CAD build for the part. Positions are in the model's coordinates, mm. Face numbers are marked on the shaded views. A direction names the side the tool comes from. Give positions to 0.01 mm unless a question says otherwise; leave off trailing zeros. Loops run counter-clockwise (first coordinate to the right, second up) from the corner with the lowest first, then second, coordinate; pieces in that order, holes last. Notation, with made-up numbers: (33.5, -8) -> (87.5, -8) arc R17 cw to (87.5, 5) -> close; hole circle Ø1 at (69, 15). An arc over 180 degrees is marked (long way). Use one line per item in the form item = value.
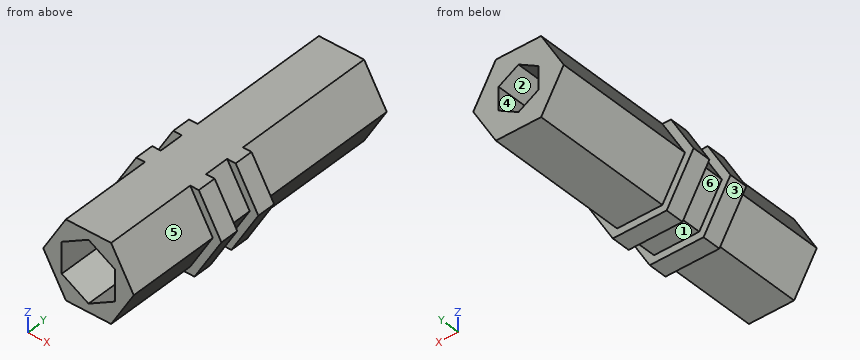
Autodesk Inventor part; units mm, degrees
ref_plane "YZ Plane" through (0, 0, 0) normal (1, 0, 0) x (0, 1, 0)
ref_plane "XZ Plane" through (0, 0, 0) normal (0, 1, 0) x (-1, 0, 0)
ref_plane "XY Plane" through (0, 0, 0) normal (0, 0, 1) x (1, 0, 0)
sketch "Sketch2" plane through (0, 0, 0) normal (0, 1, 0) x (-1, 0, 0)
  line L0 (3.6373, 0) -> (1.8187, -3.15)
  line L1 (1.8187, -3.15) -> (-1.8187, -3.15)
  line L2 (-1.8187, -3.15) -> (-3.6373, 0)
  line L3 (-3.6373, 0) -> (-1.8187, 3.15)
  line L4 (-1.8187, 3.15) -> (1.8187, 3.15)
  line L5 (1.8187, 3.15) -> (3.6373, 0)
  point P0 (0, 0)
  point P1 (0, 0)
  dimension "d0" = 6.3
extrude "Joint End" add sketch "Sketch2" along normal blind 7.5
sketch "Sketch3" plane through (0, 7.5, 0) normal (0, 1, 0) x (1, 0, 0)
  line L0 (4.3301, 0) -> (2.1651, -3.75)
  line L1 (2.1651, -3.75) -> (-2.1651, -3.75)
  line L2 (-2.1651, -3.75) -> (-4.3301, 0)
  line L3 (-4.3301, 0) -> (-2.1651, 3.75)
  line L4 (-2.1651, 3.75) -> (2.1651, 3.75)
  line L5 (2.1651, 3.75) -> (4.3301, 0)
  point P0 (0, 0)
  point P1 (0, 0)
  dimension "d3" = 7.5
extrude "Spring Stop 1" add sketch "Sketch3" along normal blind 1.5
sketch "Sketch4" plane through (0, 9, 0) normal (0, 1, 0) x (1, 0, 0)
  line L0 (3.6373, 0) -> (1.8187, -3.15)
  line L1 (1.8187, -3.15) -> (-1.8187, -3.15)
  line L2 (-1.8187, -3.15) -> (-3.6373, 0)
  line L3 (-3.6373, 0) -> (-1.8187, 3.15)
  line L4 (-1.8187, 3.15) -> (1.8187, 3.15)
  line L5 (1.8187, 3.15) -> (3.6373, 0)
  point P0 (0, 0)
  point P1 (0, 0)
  point P2 (0, 0)
  dimension "d6" = 6.3
extrude "Spring Slot" add sketch "Sketch4" along normal blind 2
sketch "Sketch5" plane through (0, 11, 0) normal (0, 1, 0) x (1, 0, 0)
  line L0 (4.3301, 0) -> (2.1651, -3.75)
  line L1 (2.1651, -3.75) -> (-2.1651, -3.75)
  line L2 (-2.1651, -3.75) -> (-4.3301, 0)
  line L3 (-4.3301, 0) -> (-2.1651, 3.75)
  line L4 (-2.1651, 3.75) -> (2.1651, 3.75)
  line L5 (2.1651, 3.75) -> (4.3301, 0)
  point P0 (0, 0)
  point P1 (0, 0)
  dimension "d9" = 7.5
extrude "Spring Stop 2" add sketch "Sketch5" along normal blind 1.5
sketch "Sketch6" plane through (0, 12.5, 0) normal (0, 1, 0) x (1, 0, 0)
  line L0 (3.6373, 0) -> (1.8187, -3.15)
  line L1 (1.8187, -3.15) -> (-1.8187, -3.15)
  line L2 (-1.8187, -3.15) -> (-3.6373, 0)
  line L3 (-3.6373, 0) -> (-1.8187, 3.15)
  line L4 (-1.8187, 3.15) -> (1.8187, 3.15)
  line L5 (1.8187, 3.15) -> (3.6373, 0)
  point P0 (0, 0)
  point P1 (0, 0)
  dimension "d12" = 6.3
extrude "Carbon End" add sketch "Sketch6" along normal blind 11.5
sketch "Sketch10" plane through (0, 0, 0) normal (0, -1, 0) x (1, 0, 0)
  line L0 (0, -2.4826) -> (-2.15, -1.2413)
  line L1 (-2.15, -1.2413) -> (-2.15, 1.2413)
  line L2 (-2.15, 1.2413) -> (0, 2.4826)
  line L3 (0, 2.4826) -> (2.15, 1.2413)
  line L4 (2.15, 1.2413) -> (2.15, -1.2413)
  line L5 (2.15, -1.2413) -> (0, -2.4826)
  point P0 (0, 0)
  point P1 (0, 0)
  dimension "d27" = 4.3
extrude "Arm Hole" cut sketch "Sketch10" against normal blind 10
sketch "Sketch11" plane through (0, 24, 0) normal (0, 1, 0) x (1, 0, 0)
  line L0 (0, -1.8475) -> (-1.6, -0.9238)
  line L1 (-1.6, -0.9238) -> (-1.6, 0.9238)
  line L2 (-1.6, 0.9238) -> (0, 1.8475)
  line L3 (0, 1.8475) -> (1.6, 0.9238)
  line L4 (1.6, 0.9238) -> (1.6, -0.9238)
  line L5 (1.6, -0.9238) -> (0, -1.8475)
  point P0 (0, 0)
  point P1 (0, 0)
  dimension "d30" = 3.2
  dimension "d31" = 3.695
extrude "Carbon Hole" cut sketch "Sketch11" against normal blind 10
sketch "Sketch12" plane through (0, 12.5, 0) normal (0, 1, 0) x (1, 0, 0)
  line L0 (2.1651, -3.75) -> (4.3301, 0)
  line L1 (-4.3301, 0) -> (-2.1651, -3.75)
  line L2 (-2.1651, -3.75) -> (2.1651, -3.75)
  line L3 (-2.5115, -3.15) -> (2.5115, -3.15)
  line L4 (2.5115, -3.15) -> (2.1651, -3.75)
  line L5 (2.1651, -3.75) -> (-2.1651, -3.75)
  line L6 (-2.1651, -3.75) -> (-2.5115, -3.15)
  point P0 (0, 0)
extrude "Bottom Cutout" cut sketch "Sketch12" against normal blind 5
properties part number "3DR-Rod-Adapter-Enlightx-v2"
1. Cut at B-B, the plane y = 17.25. Write the cut outline in (x, z), then the cut area to 3 significant figures.
Result sheet:
outline = (-3.64, 0) -> (-1.82, -3.15) -> (1.82, -3.15) -> (3.64, 0) -> (1.82, 3.15) -> (-1.82, 3.15) -> close; hole (-1.6, -0.92) -> (0, -1.85) -> (1.6, -0.92) -> (1.6, 0.92) -> (0, 1.85) -> (-1.6, 0.92) -> close
area = 25.5 mm^2
2. Mould opens along X. For the marked faces 1, 2 and 3 say: pulls with the +X half, pulls with the -X half, needs draft (parallel to the pull), parting line crosses it, or undercut.
Result sheet:
face_1 = needs draft
face_2 = undercut
face_3 = pulls with the -X half
3. Tool access for the marked faces 4, 5 and 6: list every direction of +Z, -Z, +X, -X, +Y, -Y with a clear straight run to the whole face (end or side of a thin tool).
Result sheet:
face_4 = +Y
face_5 = +Z, +X, -Y
face_6 = -Z, -X
4. Cut at D-D, the plane z = -1.5. Write the cut outline in (x, y), then the cut area to 3 significant figures.
Result sheet:
outline = (-3.46, 7.5) -> (-2.77, 7.5) -> (-2.77, 0) -> (-1.7, 0) -> (-1.7, 10) -> (1.7, 10) -> (1.7, 0) -> (2.77, 0) -> (2.77, 7.5) -> (3.46, 7.5) -> (3.46, 9) -> (2.77, 9) -> (2.77, 11) -> (3.46, 11) -> (3.46, 12.5) -> (2.77, 12.5) -> (2.77, 24) -> (0.6, 24) -> (0.6, 14) -> (-0.6, 14) -> (-0.6, 24) -> (-2.77, 24) -> (-2.77, 12.5) -> (-3.46, 12.5) -> (-3.46, 11) -> (-2.77, 11) -> (-2.77, 9) -> (-3.46, 9) -> close
area = 91.1 mm^2
5. Cut at A-A, the plane y = 8.5. Write the cut outline in (x, z).
Result sheet:
outline = (-4.33, 0) -> (-2.17, -3.75) -> (2.17, -3.75) -> (4.33, 0) -> (2.51, 3.15) -> (-2.51, 3.15) -> close; hole (-2.15, -1.24) -> (0, -2.48) -> (2.15, -1.24) -> (2.15, 1.24) -> (0, 2.48) -> (-2.15, 1.24) -> close
6. Cut at C-C, the plane x = 1.25. Write the cut outline in (y, z), then the cut area to 3 significant figures.
Result sheet:
outline = (0, -3.15) -> (7.5, -3.15) -> (7.5, -3.75) -> (9, -3.75) -> (9, -3.15) -> (11, -3.15) -> (11, -3.75) -> (12.5, -3.75) -> (12.5, -3.15) -> (24, -3.15) -> (24, -1.13) -> (14, -1.13) -> (14, 1.13) -> (24, 1.13) -> (24, 3.15) -> (0, 3.15) -> (0, 1.76) -> (10, 1.76) -> (10, -1.76) -> (0, -1.76) -> close
area = 95.3 mm^2
7. Drill centre lines: line 1 (Y direction, x = 3.5, z = 0.5); line 2 (X direction, y = 6, z = -0.25); line 3 (Z direction, x = 1, y = 9.5). Where is each one in solid material? Low to high.
Result sheet:
line_1 = 7.5 to 9, 11 to 12.5
line_2 = -3.49 to -2.15, 2.15 to 3.49
line_3 = -3.15 to -1.91, 1.91 to 3.15
8. Drop flat-ended pins along their axis: P1, Ø1, axis at y = 4, z = 1, coming from the -X side; P2, Ø1.1, axis at x = 0, y = 18.5, coming from the -Z side; P3, Ø2, axis at y = 19.5, z = 0, coming from the +X side. Give the stop position or say it passes through.
Result sheet:
P1 = -3.35
P2 = -3.15
P3 = 3.64
